Here's how the part is built. I have some questions about the finished solid (model axes, mm). A direction names the side the tool comes from. Round coordinates to 2 decimals unless told otherwise and drop trailing zeros. Write each loop counter-clockwise with the first axis right and the second up, starting at its lowest first coordinate (ties: lowest second). Pieces come first, ordered by that corner, then holes. Notation, with made-up numbers: (-24.5, -9) -> (-11.5, -9) arc R27 ccw to (-11.5, 17) -> close; hole circle Ø7 at (71, -0.5). An arc over 180 degrees is marked (long way). Answer as CSV lines item,"result".
```python
from build123d import *

# Parameters (mm, degrees)
PAD_DEPTH       = 77.5
SKETCH001_R     = 2.5
POCKET_DEPTH    = 6
CHAMFER_SIZE    = 1
SKETCH002_R     = 3
POCKET001_DEPTH = 6


with BuildPart() as part:
    # Sketch → Pad (new body)
    with BuildSketch(Plane.XZ):
        Polygon((-22, 30), (22, 30), (22, 4.6), (10, 4.6), (10, 17.5), (-10, 17.5), (-10, 4.6), (-22, 4.6), align=None)
    extrude(amount=PAD_DEPTH)

    # Sketch001 (on Face3 of Pad) → Pocket (cut)
    with BuildSketch(Plane(origin=(0, 0, 30), x_dir=(-1, 0, 0), z_dir=(0, 0, 1))):
        with Locations((-16, 20.75)):
            Circle(SKETCH001_R)
        with Locations((16, 20.75)):
            Circle(SKETCH001_R)
        with Locations((16, 56.75)):
            Circle(SKETCH001_R)
        with Locations((-16, 56.75)):
            Circle(SKETCH001_R)
    extrude(amount=-POCKET_DEPTH, mode=Mode.SUBTRACT)

    # Chamfer
    chamfer_edges = [part.edges().sort_by_distance(p)[0] for p in [
        (22, -38.75, 4.6),
        (22, -38.75, 30),
        (-22, -38.75, 30),
        (-22, -38.75, 4.6),
        (-10, -38.75, 4.6),
        (10, -38.75, 4.6),
        (-10, -77.5, 11.05),
        (0, -77.5, 17.5),
        (10, -77.5, 11.05),
        (16, -77.5, 4.6),
        (22, -77.5, 17.3),
        (0, -77.5, 30),
        (-22, -77.5, 17.3),
        (-10, 0, 11.05),
        (-16, 0, 4.6),
        (-22, 0, 17.3),
        (0, 0, 30),
        (22, 0, 17.3),
        (16, 0, 4.6),
        (10, 0, 11.05),
        (0, 0, 17.5),
        (-16, -77.5, 4.6),
    ]]
    chamfer(chamfer_edges, length=CHAMFER_SIZE)

    # Sketch002 → Pocket001 (cut)
    with BuildSketch(Plane.XZ):
        with Locations((0, 24)):
            Circle(SKETCH002_R)
    extrude(amount=POCKET001_DEPTH, mode=Mode.SUBTRACT)


solid = part.part
```
1. Suppose I cut it at C-C on y = -20.75. Please give me the cut outline in (x, z), and give its area (3 significant figures).
Numbers:
outline,"(-22, 5.6) -> (-21, 4.6) -> (-11, 4.6) -> (-10, 5.6) -> (-10, 17.5) -> (10, 17.5) -> (10, 5.6) -> (11, 4.6) -> (21, 4.6) -> (22, 5.6) -> (22, 29) -> (21, 30) -> (18.5, 30) -> (18.5, 24) -> (13.5, 24) -> (13.5, 30) -> (-13.5, 30) -> (-13.5, 24) -> (-18.5, 24) -> (-18.5, 30) -> (-21, 30) -> (-22, 29) -> close"
area,"797 mm^2"
2. If we mould it in two halves opening along X, with no side actions, what happens to faces 1 (the face through (22, -38, 17)), 2 (the face through (-13.502, -56.86, 27.042)), 3 (the face through (-16, -38, 4.6))? For each: released by +X, released by -X, zero draft, split by the parting line, or undercut.
Numbers:
face 1,"released by +X"
face 2,"undercut"
face 3,"zero draft"
3. Suppose I cut it at A-A on z = 27.75. Please give me the cut outline in (x, y), and give its area (3 significant figures).
Numbers:
outline,"(-22, -76.5) -> (-21, -77.5) -> (21, -77.5) -> (22, -76.5) -> (22, -1) -> (21, 0) -> (-21, 0) -> (-22, -1) -> close; hole circle Ø5 at (-16, -56.75); hole circle Ø5 at (-16, -20.75); hole circle Ø5 at (16, -56.75); hole circle Ø5 at (16, -20.75)"
area,"3,330 mm^2"
4. If I drill on line 1 (X direction, y = -20.75, z = 28.2); line 2 (Y direction, x = 16, z = 26.3); line 3 (X direction, y = -47.5, z = 9.5), over which ranges is the centre line in solid material (lowest first)?
Numbers:
line 1,"x = -22 to -18.5, -13.5 to 13.5, 18.5 to 22"
line 2,"y = -77.5 to -59.25, -54.25 to -23.25, -18.25 to 0"
line 3,"x = -22 to -10, 10 to 22"
5. For pin 1 Ø3 at (x, y) = (-16, -20.75) entering from +Z; pin 2 Ø16 at (x, y) = (1, -40) entering from -Z; pin 3 Ø1.8 at (x, z) = (1, 25.5) entering from +Y; pin 4 Ø6 at (x, z) = (-2, 14) entering from +Y, each with a flat end and sliding along its axis, tell me the tip position at first contact or that it passes through.
Numbers:
pin 1,"stops at z = 24"
pin 2,"stops at z = 17.5"
pin 3,"stops at y = -6"
pin 4,"passes through"
6. Suppose I cut it at D-D on x = -14.5. Please give me the cut outline in (y, z), and give its area (3 significant figures).
Numbers:
outline,"(-77.5, 5.6) -> (-76.5, 4.6) -> (-1, 4.6) -> (0, 5.6) -> (0, 29) -> (-1, 30) -> (-18.75, 30) -> (-18.75, 24) -> (-22.75, 24) -> (-22.75, 30) -> (-54.75, 30) -> (-54.75, 24) -> (-58.75, 24) -> (-58.75, 30) -> (-76.5, 30) -> (-77.5, 29) -> close"
area,"1,920 mm^2"
7. On a 3-axis mill with a long thin cutter (end or side, diameter ignored), from which of +Z, -Z, +X, -X, +Y, -Y can I reach the whole of each face in a straight line? I mean faces 4 (the face through (18.498, -56.86, 27.042)), 5 (the face through (-0.65, -2.96, 21.07)), 6 (the face through (16, -38, 4.6)), 7 (the face through (10, -38, 11)). Say none if no direction works.
Numbers:
face 4,"+Z"
face 5,"+Y"
face 6,"-Z, +X, -X, +Y, -Y"
face 7,"-Z, +Y, -Y"
8. Suppose I cut it at B-B on z = 8.25. Please give me the cut outline in (x, y), and give its area (3 significant figures).
Numbers:
outline,"(-22, -76.5) -> (-21, -77.5) -> (-11, -77.5) -> (-10, -76.5) -> (-10, -1) -> (-11, 0) -> (-21, 0) -> (-22, -1) -> close; (10, -76.5) -> (11, -77.5) -> (21, -77.5) -> (22, -76.5) -> (22, -1) -> (21, 0) -> (11, 0) -> (10, -1) -> close"
area,"1,860 mm^2"
